For this review, take the finished solid that the model builds, in its own axes (mm). A direction names the side the tool comes from. Give positions to 0.01 mm unless a question says otherwise; leave off trailing zeros. Loops run counter-clockwise (first coordinate to the right, second up) from the corner with the lowest first, then second, coordinate; pieces in that order, holes last.
```python
from build123d import *

# Parameters (mm, degrees)
SKETCH2_W           = 40
SKETCH2_H           = 20
BOSS_EXTRUDE1_DEPTH = 2
SKETCH3_W           = 25
SKETCH3_H           = 16
BOSS_EXTRUDE2_DEPTH = 8
CUT_EXTRUDE1_DEPTH  = 10
SKETCH5_R           = 1.6
CUT_EXTRUDE2_DEPTH  = 10
SKETCH6_R           = 1.5
CUT_EXTRUDE3_DEPTH  = 30


with BuildPart() as part:
    # Sketch2 → Boss-Extrude1 (new body)
    with BuildSketch(Plane(origin=(0, 0, 0), x_dir=(1, 0, 0), z_dir=(0, 1, 0))):
        with Locations((2.363636364, -3.454545455)):
            Rectangle(SKETCH2_W, SKETCH2_H)
    extrude(amount=BOSS_EXTRUDE1_DEPTH)

    # Sketch3 → Boss-Extrude2 (add)
    with BuildSketch(Plane.XZ):
        with Locations((2.363636364, 3.454545455)):
            Rectangle(SKETCH3_W, SKETCH3_H)
    extrude(amount=-BOSS_EXTRUDE2_DEPTH)

    # Sketch1 → Cut-Extrude1 (cut)
    with BuildSketch(Plane(origin=(0, 0, 0), x_dir=(1, 0, 0), z_dir=(0, 1, 0))):
        Polygon((-7.036363636, 3.045454545), (11.763636364, 3.045454545), (11.763636364, -0.704545455), (13.113636364, -0.704545455), (13.113636364, -6.204545455), (11.763636364, -6.204545455), (11.763636364, -9.954545455), (-7.036363636, -9.954545455), (-7.036363636, -6.204545455), (-8.386363636, -6.204545455), (-8.386363636, -0.704545455), (-7.036363636, -0.704545455), align=None)
    extrude(amount=CUT_EXTRUDE1_DEPTH, mode=Mode.SUBTRACT)

    # Sketch5 → Cut-Extrude2 (cut)
    with BuildSketch(Plane.XZ):
        with Locations((18.363636364, 3.454545455)):
            Circle(SKETCH5_R)
        with Locations((-13.636363636, 3.454545455)):
            Circle(SKETCH5_R)
    extrude(amount=-CUT_EXTRUDE2_DEPTH, mode=Mode.SUBTRACT)

    # Sketch6 → Cut-Extrude3 (cut)
    with BuildSketch(Plane.XY.offset(11.454545455)):
        with Locations((2.363636364, 5)):
            Circle(SKETCH6_R)
    extrude(amount=-CUT_EXTRUDE3_DEPTH, mode=Mode.SUBTRACT)


solid = part.part
```
Item 1: The part is to be moulded in two halves that separate along X. For faces 4 (the flat face through (13.114, 4, 3)), 5 (the flat face through (2, 7, -4.545)), 6 (the flat face through (-10.136, 5, 3)), say which applies: released by +X, released by -X, zero draft, split by the parting line, or undercut.
Answer:
face 4: undercut
face 5: zero draft
face 6: released by -X
Item 2: Clearance check with flat-ended pins moving along their axes: pin 1 Ø1.1 at (y, z) = (5, 9) entering from -X; pin 2 Ø2.5 at (x, y) = (4, 5.5) entering from +Z; pin 3 Ø2.5 at (x, y) = (2.36, 5) entering from +Z; pin 4 Ø3 at (y, z) = (5, -0.5) entering from +X. State where each tip first meets the part, or that it passes through.
Answer:
pin 1: stops at x = -10.14
pin 2: stops at z = 11.45
pin 3: passes through
pin 4: stops at x = 14.86
Item 3: Take a section at D-D on y = 3. Give the boundary of the cut face in (x, z).
Answer:
outline: (-10.14, -4.55) - (14.86, -4.55) - (14.86, 11.45) - (-10.14, 11.45) - close; hole (-8.39, 0.7) - (-7.04, 0.7) - (-7.04, -3.05) - (11.76, -3.05) - (11.76, 0.7) - (13.11, 0.7) - (13.11, 6.2) - (11.76, 6.2) - (11.76, 9.95) - (-7.04, 9.95) - (-7.04, 6.2) - (-8.39, 6.2) - close
Item 4: Take a section at B-B on y = 5. Give the boundary of the cut face in (x, z).
Answer:
outline: (-10.14, -4.55) - (0.86, -4.55) - (0.86, -3.05) - (-7.04, -3.05) - (-7.04, 0.7) - (-8.39, 0.7) - (-8.39, 6.2) - (-7.04, 6.2) - (-7.04, 9.95) - (0.86, 9.95) - (0.86, 11.45) - (-10.14, 11.45) - close; (3.86, -4.55) - (14.86, -4.55) - (14.86, 11.45) - (3.86, 11.45) - (3.86, 9.95) - (11.76, 9.95) - (11.76, 6.2) - (13.11, 6.2) - (13.11, 0.7) - (11.76, 0.7) - (11.76, -3.05) - (3.86, -3.05) - close
Item 5: Tool access review of faces 1 (the flat face through (14.864, 5, 3)), 2 (the flat face through (-8, 4, 0.705)), 3 (the flat face through (2, 7, 11.455)): name each direction out of +Z, -Z, +X, -X, +Y, -Y from which nothing blocks a thin tool from reaching the whole face with its end or side.
Answer:
face 1: +Z, -Z, +X, +Y
face 2: +Y, -Y
face 3: +Z, +X, -X, +Y
Item 6: For L1, parallel to Z at x = 4.5, y = 4; L2, parallel to X at y = 3.25, z = 9; L3, parallel to X at y = 4, z = 1.5, list the stretches that pass through material, from the lowest coordinate up.
Answer:
L1: z = -4.55 to -3.05, 9.95 to 11.45
L2: x = -10.14 to -7.04, 11.76 to 14.86
L3: x = -10.14 to -8.39, 13.11 to 14.86
Item 7: Take a section at A-A on x = 8. Give the boundary of the cut face in (y, z).
Answer:
outline: (0, -6.55) - (2, -6.55) - (2, -4.55) - (8, -4.55) - (8, -3.05) - (0, -3.05) - close; (0, 9.95) - (8, 9.95) - (8, 11.45) - (2, 11.45) - (2, 13.45) - (0, 13.45) - close
Item 8: Take a section at C-C on z = 7.75. Give the boundary of the cut face in (x, y), and give its area (3 significant figures).
Answer:
outline: (-17.64, 0) - (-7.04, 0) - (-7.04, 8) - (-10.14, 8) - (-10.14, 2) - (-17.64, 2) - close; (11.76, 0) - (22.36, 0) - (22.36, 2) - (14.86, 2) - (14.86, 8) - (11.76, 8) - close
area: 79.6 mm2
